from build123d import *

# Parameters (mm, degrees)
F1_DEPTH  = 2311.4
F3_DEPTH  = 2311.4
F4_DEPTH  = 2311.4
F2_W      = 1117.6
F2_H      = 25.4
F9_DEPTH  = 50.8
F7_W      = 571.5
F7_H      = 25.4
F10_DEPTH = 50.8
F8_W      = 571.5
F8_H      = 25.4
F11_DEPTH = 50.8
F12_W     = 571.5
F12_H     = 25.4
F13_DEPTH = 203.2
F14_W     = 571.5
F14_H     = 25.4
F15_DEPTH = 203.2
F16_W     = 711.2
F16_H     = 25.4
F17_DEPTH = 254


with BuildPart() as f1:
    # F0 (on Top) → F1 (new body)
    with BuildSketch(Plane.XY):
        Polygon((-558.8, 285.75), (558.8, 285.75), (584.2, 311.15), (-584.2, 311.15), align=None)
    extrude(amount=F1_DEPTH)

    # F0 (on Top) → F3 (join)
    with BuildSketch(Plane.XY):
        Polygon((-558.8, -285.75), (-558.8, 285.75), (-584.2, 311.15), (-584.2, -311.15), align=None)
    extrude(amount=F3_DEPTH)

    # F0 (on Top) → F4 (join)
    with BuildSketch(Plane.XY):
        Polygon((558.8, 285.75), (558.8, -285.75), (584.2, -311.15), (584.2, 311.15), align=None)
    extrude(amount=F4_DEPTH)

    # F2 (on face) → F9 (join)
    with BuildSketch(Plane.XZ.offset(-285.75)):
        with Locations((0, 393.7)):
            Rectangle(F2_W, F2_H)
        with Locations((0, 749.3)):
            Rectangle(F2_W, F2_H)
        with Locations((0, 1104.9)):
            Rectangle(F2_W, F2_H)
        with Locations((0, 1460.5)):
            Rectangle(F2_W, F2_H)
    extrude(amount=F9_DEPTH)

    # F7 (on face) → F10 (join)
    with BuildSketch(Plane.YZ.offset(-558.8)):
        with Locations((0, 1460.5)):
            Rectangle(F7_W, F7_H)
        with Locations((0, 1104.9)):
            Rectangle(F7_W, F7_H)
        with Locations((0, 749.3)):
            Rectangle(F7_W, F7_H)
        with Locations((0, 393.7)):
            Rectangle(F7_W, F7_H)
    extrude(amount=F10_DEPTH)

    # F8 (on face) → F11 (join)
    with BuildSketch(Plane(origin=(558.8, 0, 0), x_dir=(0, -1, 0), z_dir=(-1, 0, 0))):
        with Locations((0, 393.7)):
            Rectangle(F8_W, F8_H)
        with Locations((0, 749.3)):
            Rectangle(F8_W, F8_H)
        with Locations((0, 1104.9)):
            Rectangle(F8_W, F8_H)
        with Locations((0, 1460.5)):
            Rectangle(F8_W, F8_H)
    extrude(amount=F11_DEPTH)

    # F12 (on face) → F13 (join)
    with BuildSketch(Plane.YZ.offset(-558.8)):
        with Locations((0, 419.1)):
            Rectangle(F12_W, F12_H)
        with Locations((0, 774.7)):
            Rectangle(F12_W, F12_H)
        Polygon((234.95, 1117.6), (285.75, 1117.6), (285.75, 1143), (-285.75, 1143), (-285.75, 1117.6), align=None)
        with Locations((0, 1485.9)):
            Rectangle(F12_W, F12_H)
    extrude(amount=F13_DEPTH)

    # F14 (on face) → F15 (join)
    with BuildSketch(Plane(origin=(558.8, 0, 0), x_dir=(0, -1, 0), z_dir=(-1, 0, 0))):
        with Locations((0, 1485.9)):
            Rectangle(F14_W, F14_H)
        with Locations((0, 774.7)):
            Rectangle(F14_W, F14_H)
        with Locations((0, 419.1)):
            Rectangle(F14_W, F14_H)
        with Locations((0, 1130.3)):
            Rectangle(F14_W, F14_H)
    extrude(amount=F15_DEPTH)

    # F16 (on face) → F17 (join)
    with BuildSketch(Plane.XZ.offset(-285.75)):
        with Locations((0, 419.1)):
            Rectangle(F16_W, F16_H)
        with Locations((0, 1485.9)):
            Rectangle(F16_W, F16_H)
        with Locations((0, 774.7)):
            Rectangle(F16_W, F16_H)
        with Locations((0, 1130.3)):
            Rectangle(F16_W, F16_H)
    extrude(amount=F17_DEPTH)


solid = f1.part
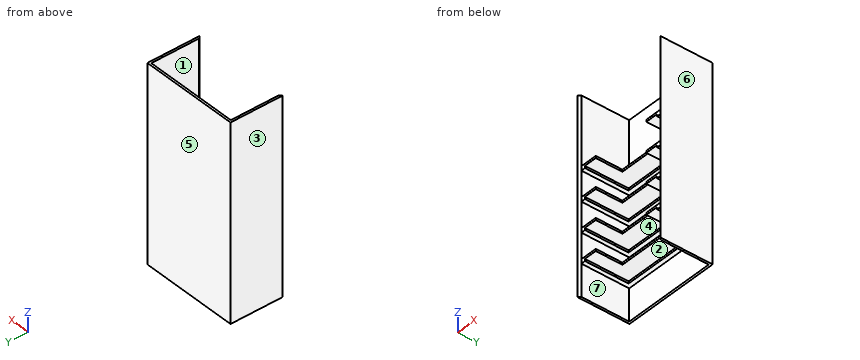
Could you check a few things on this model? Use its own coordinates, in mm. Face numbers are marked on the shaded views. A direction names the side the tool comes from. Coordinates: 2 decimals unless noted, no trailing zeros. Write each loop counter-clockwise with the first axis right and the second up, starting at its lowest first coordinate (ties: lowest second). Pieces come first, ordered by that corner, then holes. Notation, with made-up numbers: M 73.25,-20 L 127.25,-20 A31 ccw 127.25,16 Z; hole C 7.25,85 d11. An arc over 180 degrees is marked long. One line per question, with ' | ' between items.
1) Imagine slicing it at C-C, the plane x = -436. Write out the boundary of the cut face in (y, z), and give its area (3 significant figures).
Checks:
outline: M -285.75,406.4 L 234.95,406.4 L 234.95,381 L 285.75,381 L 285.75,0 L 311.15,0 L 311.15,2311.4 L 285.75,2311.4 L 285.75,1498.6 L -285.75,1498.6 L -285.75,1473.2 L 234.95,1473.2 L 234.95,1447.8 L 285.75,1447.8 L 285.75,1143 L -285.75,1143 L -285.75,1117.6 L 234.95,1117.6 L 234.95,1092.2 L 285.75,1092.2 L 285.75,787.4 L -285.75,787.4 L -285.75,762 L 234.95,762 L 234.95,736.6 L 285.75,736.6 L 285.75,431.8 L -285.75,431.8 Z | area: 122,000 mm²
2) Imagine slicing it at B-B, the plane z = 2038. Write out the boundary of the cut face in (x, y).
Checks:
outline: M -584.2,-311.15 L -558.8,-285.75 L -558.8,285.75 L 558.8,285.75 L 558.8,-285.75 L 584.2,-311.15 L 584.2,311.15 L -584.2,311.15 Z
3) I need wall thicknesses on probe 1 along Z at (x, y) = (515, -56); probe 2 along Z at (x, y) = (-160, 72); probe 3 along X at (y, z) = (128, 928). Which ranges of each line are inside material? Lowest first, please. Write a range as [from, to].
Checks:
probe 1: [381, 431.8], [736.6, 787.4], [1092.2, 1143], [1447.8, 1498.6] | probe 2: [406.4, 431.8], [762, 787.4], [1117.6, 1143], [1473.2, 1498.6] | probe 3: [-584.2, -558.8], [558.8, 584.2]
4) For pin 1 Ø4 at (x, y) = (-355.5, -68.5) entering from -Z; pin 2 Ø4 at (x, z) = (-340, 789) entering from -Y; pin 3 Ø20.5 at (x, z) = (-164, 387.5) entering from -Y, each with a flat end and sliding along its axis, tell me the tip position at first contact or that it passes through.
Checks:
pin 1: z = 406.4 | pin 2: y = 31.75 | pin 3: y = 234.95
5) If we mould it in two halves opening along X, with no side actions, what happens to the marked faces 5, 6 and 7? For each: released by +X, released by -X, zero draft, split by the parting line, or undercut.
Checks:
face 5: zero draft | face 6: released by +X | face 7: undercut
6) For the marked faces 1, 2, 3 and 4, which set-ups out of +Z, -Z, +X, -X, +Y, -Y let a thin tool reach every point of the face, with its end or its side?
Checks:
face 1: +Z, -Y | face 2: -Z, -Y | face 3: +Z, -Z, -X, +Y, -Y | face 4: -Y
7) Imagine slicing it at A-A, the plane x = 14.5. Write out the boundary of the cut face in (y, z), and give its area (3 significant figures).
Checks:
outline: M 31.75,406.4 L 234.95,406.4 L 234.95,381 L 285.75,381 L 285.75,0 L 311.15,0 L 311.15,2311.4 L 285.75,2311.4 L 285.75,1498.6 L 31.75,1498.6 L 31.75,1473.2 L 234.95,1473.2 L 234.95,1447.8 L 285.75,1447.8 L 285.75,1143 L 31.75,1143 L 31.75,1117.6 L 234.95,1117.6 L 234.95,1092.2 L 285.75,1092.2 L 285.75,787.4 L 31.75,787.4 L 31.75,762 L 234.95,762 L 234.95,736.6 L 285.75,736.6 L 285.75,431.8 L 31.75,431.8 Z | area: 89,700 mm²
